```python
from build123d import *
from build123d.topology import SkipClean

# Parameters (mm, degrees)
SKETCH1_R               = 140
SKETCH1_R_2             = 97
BOSS_EXTRUDE1_DEPTH     = 225
SKETCH5_R               = 23.5
BOSS_EXTRUDE2_DEPTH     = 32
CIRPATTERN1_COUNT       = 3
MIRROR1_COPY_1_SKETCH_R = 23.5
MIRROR1_COPY_1_DEPTH    = 32
MIRROR1_COPY_2_SKETCH_R = 23.5
MIRROR1_COPY_2_DEPTH    = 32
BOSS_EXTRUDE3_START     = -42.02041
SKETCH6_R               = 100
BOSS_EXTRUDE3_DEPTH     = 42.02041
SKETCH7_R               = 50
CUT_EXTRUDE1_DEPTH      = 25
SKETCH8_R               = 28
CUT_EXTRUDE2_DEPTH      = 455.845123838
SKETCH9_R               = 12
CUT_EXTRUDE3_DEPTH      = 15
CIRPATTERN2_COUNT       = 3


with BuildPart() as part:
    # Sketch1 → Boss-Extrude1 (new body)
    with BuildSketch(Plane(origin=(0, 0, 0), x_dir=(1, 0, 0), z_dir=(0, 1, 0))):
        with Locations(Location((0, 0, 0), (0, 0, 270))):
            Circle(SKETCH1_R)
        with Locations(Location((0, 0, 0), (0, 0, 270))):
            Circle(SKETCH1_R_2, mode=Mode.SUBTRACT)
    extrude(amount=BOSS_EXTRUDE1_DEPTH)

    # Sketch5 → Boss-Extrude2 (add)
    with BuildSketch(Plane(origin=(0, 0, 0), x_dir=(-1, 0, 0), z_dir=(0, -1, 0))):
        with BuildLine():
            ThreePointArc((50, 176.795082097), (0, 225.032212821), (-50, 176.795082097))
            Line((-50, 176.795082097), (-50, 173.204917903))
            Line((-50, 173.204917903), (-50, 130.766968306))
            ThreePointArc((-50, 130.766968306), (0, 140), (50, 130.766968306))
            Line((50, 130.766968306), (50, 173.204917903))
            Line((50, 173.204917903), (50, 176.795082097))
        make_face()
        with Locations(Location((0, 175, 0), (0, 0, 90))):
            Circle(SKETCH5_R, mode=Mode.SUBTRACT)
    boss_extrude2 = extrude(amount=-BOSS_EXTRUDE2_DEPTH)

    # CirPattern1: Boss-Extrude2 ×3 about axis
    cirpattern1_axis = Axis((0, 0, 0), (0, 1, 0))
    for i in range(1, CIRPATTERN1_COUNT):
        add(boss_extrude2.rotate(cirpattern1_axis, i * 360 / CIRPATTERN1_COUNT))

    # Mirror1: Boss-Extrude2 across plane
    add(boss_extrude2.mirror(Plane(origin=(0, 112.5, 0), x_dir=(0, 0, 1), z_dir=(0, -1, 0))))

    # Mirror1 copy 1 sketch → Mirror1 copy 1 (add)
    with BuildSketch(Plane(origin=(0, 225, 0), x_dir=(0.4999999999999998, 0, 0.8660254037844387), z_dir=(0, 1, 0))):
        with BuildLine():
            ThreePointArc((50, -176.795082097), (0, -225.032212821), (-50, -176.795082097))
            Line((-50, -176.795082097), (-50, -173.204917903))
            Line((-50, -173.204917903), (-50, -130.766968306))
            ThreePointArc((-50, -130.766968306), (0, -140), (50, -130.766968306))
            Line((50, -130.766968306), (50, -173.204917903))
            Line((50, -173.204917903), (50, -176.795082097))
        make_face()
        with Locations((0, -175)):
            Circle(MIRROR1_COPY_1_SKETCH_R, mode=Mode.SUBTRACT)
    extrude(amount=-MIRROR1_COPY_1_DEPTH)

    # Mirror1 copy 2 sketch → Mirror1 copy 2 (add)
    with BuildSketch(Plane(origin=(0, 225, 0), x_dir=(0.5000000000000004, 0, -0.8660254037844384), z_dir=(0, 1, 0))):
        with BuildLine():
            ThreePointArc((50, -176.795082097), (0, -225.032212821), (-50, -176.795082097))
            Line((-50, -176.795082097), (-50, -173.204917903))
            Line((-50, -173.204917903), (-50, -130.766968306))
            ThreePointArc((-50, -130.766968306), (0, -140), (50, -130.766968306))
            Line((50, -130.766968306), (50, -173.204917903))
            Line((50, -173.204917903), (50, -176.795082097))
        make_face()
        with Locations((0, -175)):
            Circle(MIRROR1_COPY_2_SKETCH_R, mode=Mode.SUBTRACT)
    extrude(amount=-MIRROR1_COPY_2_DEPTH)

    # Sketch6 → Boss-Extrude3 (add)
    with SkipClean():  # the faces are left unmerged after this step: merging them gives an invalid solid
        with BuildSketch(Plane.XY.offset(140).offset(BOSS_EXTRUDE3_START)):
            with Locations((0, 112.5)):
                Circle(SKETCH6_R)
        extrude(amount=BOSS_EXTRUDE3_DEPTH)

    # Sketch7 → Cut-Extrude1 (cut)
    with SkipClean():  # the faces are left unmerged after this step: merging them gives an invalid solid
        with BuildSketch(Plane.XY.offset(140)):
            with Locations((0, 112.5)):
                Circle(SKETCH7_R)
        extrude(amount=-CUT_EXTRUDE1_DEPTH, mode=Mode.SUBTRACT)

    # Sketch8 → Cut-Extrude2 (cut, through all)
    with SkipClean():  # the faces are left unmerged after this step: merging them gives an invalid solid
        with BuildSketch(Plane.XY.offset(115)):
            with Locations((0, 112.5)):
                Circle(SKETCH8_R)
        extrude(amount=-CUT_EXTRUDE2_DEPTH, mode=Mode.SUBTRACT)

    # Sketch9 → Cut-Extrude3 (cut)
    with SkipClean():  # the faces are left unmerged after this step: merging them gives an invalid solid
        with BuildSketch(Plane.XY.offset(140)):
            with Locations((0, 187.5)):
                Circle(SKETCH9_R)
        cut_extrude3 = extrude(amount=-CUT_EXTRUDE3_DEPTH, mode=Mode.SUBTRACT)

    # CirPattern2: Cut-Extrude3 ×3 about axis
    with SkipClean():  # the faces are left unmerged after this step: merging them gives an invalid solid
        cirpattern2_axis = Axis((0, 112.5, 0), (0, 0, 1))
        for i in range(1, CIRPATTERN2_COUNT):
            add(cut_extrude3.rotate(cirpattern2_axis, i * 360 / CIRPATTERN2_COUNT), mode=Mode.SUBTRACT)


solid = part.part
```
Part model, mm, in its own coordinate system. A direction names the side the tool comes from. Round coordinates to 2 decimals unless told otherwise and drop trailing zeros. Write each loop counter-clockwise with the first axis right and the second up, starting at its lowest first coordinate (ties: lowest second). Pieces come first, ordered by that corner, then holes. Notation, with made-up numbers: M -39,-35.75 L 5,-35.75 A9 ccw 5,-29.75 Z; hole C 52,30 d5. An arc over 180 degrees is marked long. Answer as CSV lines item,"result". Start each with the question number.
1) Which spindle directions (+Z, -Z, +X, -X, +Y, -Y) get a long thin tool onto all of the face, cutting with end or side? Do faces 4 (the face through (-50, 209, -153)), 5 (the face through (166, 193, 108)), 6 (the face through (108.457, 15.776, 120.353)), 7 (the face through (-65, 75, 125)), 8 (the face through (-177, 193, 90)). Say none if no direction does.
2) Drill centre lines: L1, parallel to Y at x = 0, z = 130; L2, parallel to Y at x = 0, z = 108; L3, parallel to Y at x = 0, z = 124. Where is each one in solid material? Low to high.
3) Band-saw the part on B-B (x = -167). List the corners of the cut face in (y, z), then the cut area to 3 significant figures.
4) Drop flat-ended pins along their axis: pin 1 (6 mm diameter, centred on x = 123.5, y = 54, fed in from +Z); pin 2 (7 mm diameter, centred on x = 59.5, y = 79, fed in from +Z); pin 3 (6 mm diameter, centred on x = -114.5, y = 24.5, fed in from -Z). Give the stop position or say it passes through.
5) Band-saw the part on C-C (z = 87.5). Count the separate pieces of the cut face and the enclosed holes in it, then the cut area to 3 significant figures.
6) Mould opens along Y. For faces 1 (the face through (56.1, 83.1, 132.6)), 2 (the face through (-14, 0, -97)), 3 (the face through (167.44, 15.78, 104.82)) say: +Y half, -Y half, draft (parallel to the pull), parting line (faces both ways), or undercut.
7) Band-saw the part on D-D (y = 156). List the corners of the cut face in (x, z).
8) Band-saw the part on A-A (z = 0). List the corners of the cut face in (x, y), then the cut area to 4 significant figures.
Worked out:
1,face 4,"-Z, -X, +Y, -Y"
1,face 5,"+Z, +X"
1,face 6,"+Z, -Y"
1,face 7,"+Z"
1,face 8,"+Z, -X"
2,L1,"0 to 62.5, 162.5 to 175.5, 199.5 to 225"
2,L2,"0 to 84.5, 140.5 to 225"
2,L3,"0 to 62.5, 162.5 to 225"
3,outline,"M 0,38.68 L 32,38.68 L 32,69.79 L 0,69.79 Z; M 0,105.21 L 32,105.21 L 32,135.09 L 0,135.09 Z; M 193,38.68 L 225,38.68 L 225,69.79 L 193,69.79 Z; M 193,105.21 L 225,105.21 L 225,135.09 L 193,135.09 Z"
3,area,"3,900 mm²"
4,pin 1,"z = 71.27"
4,pin 2,"z = 125"
4,pin 3,"z = -84.66"
5,separate pieces,"6"
5,enclosed holes,"0"
5,area,"36,100 mm²"
6,face 1,"undercut"
6,face 2,"-Y half"
6,face 3,"draft"
7,outline,"M -90.04,107.2 A140 ccw long 90.04,107.2 L 90.04,140 L 24.65,140 L 24.65,115 L -24.65,115 L -24.65,140 L -90.04,140 Z; hole C 0,0 d194"
8,outline,"M -140,0 L -97,0 L -97,225 L -140,225 Z; M 97,0 L 140,0 L 140,225 L 97,225 Z"
8,area,"19,350 mm²"
